The model under review builds one solid part; all positions refer to its coordinate system, in mm. Face numbers are marked on the shaded views. A direction names the side the tool comes from. Round coordinates to 2 decimals unless told otherwise and drop trailing zeros. Order: outer loops, then holes, each group sorted by start corner. A loop starts at its lowest first (then second) coordinate and runs counter-clockwise, first axis right, second up.
1) Consider section C-C (y = 49). Give the boundary of the cut face in (x, z).
2) Mouldability with a two-part tool opening along X and no side actions: class the marked faces 3, 4 and 5 as pulls with the +X half, pulls with the -X half, needs draft (parallel to the pull), parting line crosses it, or undercut.
3) To check wall thickness, follow L1, parallel to X at y = 69, z = -373; L2, parallel to X at y = 66, z = 120.5; L3, parallel to Y at x = -150, z = 281. State the ranges of each line that lie inside material, in increasing order.
4) Consider section A-A (x = 88.51). Give the boundary of the cut face in (y, z), then the cut area to 3 significant figures.
5) Consider section B-B (z = -186.5). Give the boundary of the cut face in (x, y).
6) Machinability: for the marked faces 1 and 2, which of the approach directions +Z, -Z, +X, -X, +Y, -Y give a long, thin tool a straight path to every point of the face, cutting with its end or side? Answer none if there is none.
7) Clearance check with flat-ended pins moving along their axes: P1, Ø12, axis at x = -106.5, y = 73.5, coming from the +Z side; P2, Ø3, axis at x = 51.5, z = -3.5, coming from the -Y side; P3, Ø6, axis at x = 109.5, z = 313.5, coming from the -Y side; P4, Ø5, axis at x = 29.5, y = 18.5, coming from the +Z side. State where each tip first meets the part, or that it passes through.
8) Consider section D-D (x = 10). Give the boundary of the cut face in (y, z).
from build123d import *

# Parameters (mm, degrees)
BOSS_EXTRUDE1_DEPTH = 591.5
SKETCH2_W           = 388.02090207
SKETCH2_H           = 25.404192512
BOSS_EXTRUDE2_DEPTH = 232
FILLET1_R           = 12.7
FILLET3_R           = 6.35


with BuildPart() as part:
    # Sketch1 → Boss-Extrude1 (new body)
    with BuildSketch(Plane(origin=(0, 0, -411.75), x_dir=(-1, 0, 0), z_dir=(0, 0, -1))):
        with BuildLine():
            Line((121.01, 20.009665474), (194.010451035, 36.954192512))
            Line((194.010451035, 36.954192512), (194.010451035, 103.904192512))
            Line((194.010451035, 103.904192512), (-194.010451035, 103.904192512))
            Line((-194.010451035, 103.904192512), (-194.010451035, 36.954192512))
            Line((-194.010451035, 36.954192512), (-121.01, 20.009665474))
            Line((-121.01, 20.009665474), (-121.01, 39))
            ThreePointArc((-121.01, 39), (-88.51, 71.5), (-56.01, 39))
            Line((-56.01, 39), (-56.01, 5.206473282))
            ThreePointArc((-56.01, 5.206473282), (0, 0), (56.01, 5.206473282))
            Line((56.01, 5.206473282), (56.01, 39))
            ThreePointArc((56.01, 39), (88.51, 71.5), (121.01, 39))
            Line((121.01, 39), (121.01, 20.009665474))
        make_face()
    extrude(amount=-BOSS_EXTRUDE1_DEPTH)

    # Sketch2 → Boss-Extrude2 (add)
    with BuildSketch(Plane.XY.offset(179.75)):
        with Locations((0, 91.202096256)):
            Rectangle(SKETCH2_W, SKETCH2_H)
    extrude(amount=BOSS_EXTRUDE2_DEPTH)

    # Fillet1
    fillet1_edges = [part.edges().sort_by_distance(p)[0] for p in [
        (194.010451035, 70.429192512, -411.75),
        (-194.010451035, 70.429192512, -411.75),
        (194.010451035, 91.202096256, 411.75),
        (-194.010451035, 91.202096256, 411.75),
    ]]
    fillet(fillet1_edges, radius=FILLET1_R)

    # Fillet3
    fillet3_edges = [part.edges().sort_by_distance(p)[0] for p in [
        (0, 78.5, 179.75),
    ]]
    fillet(fillet3_edges, radius=FILLET3_R)


solid = part.part
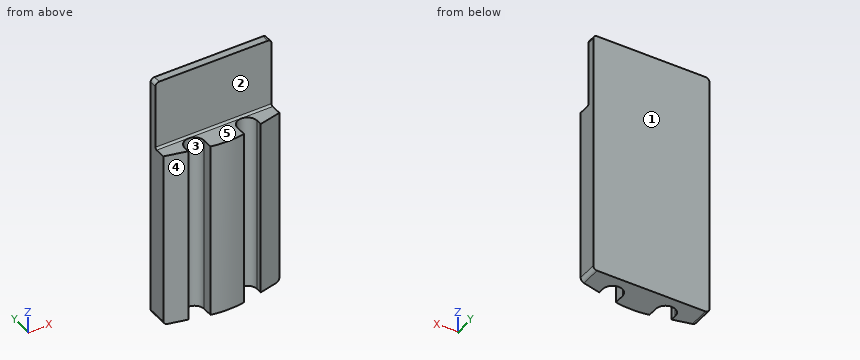
Answer below:
1. outline: (-194.01, -399.05) arc R12.7 ccw to (-181.31, -411.75) - (-119.43, -411.75) - (-119.43, 179.75) - (-194.01, 179.75) - close; (-57.59, -411.75) - (57.59, -411.75) - (57.59, 179.75) - (-57.59, 179.75) - close; (119.43, -411.75) - (181.31, -411.75) arc R12.7 ccw to (194.01, -399.05) - (194.01, 179.75) - (119.43, 179.75) - close
2. face 3: undercut
2. face 4: pulls with the -X half
2. face 5: needs draft
3. L1: x = -194.01 to -101.01, -76.01 to 76.01, 101.01 to 194.01
3. L2: x = -194.01 to -106.6, -70.42 to 70.42, 106.6 to 194.01
3. L3: y = 78.5 to 103.9
4. outline: (71.5, -411.75) - (103.9, -411.75) - (103.9, 411.75) - (78.5, 411.75) - (78.5, 186.1) arc R6.35 cw to (72.15, 179.75) - (71.5, 179.75) - close
4. area: 25,100 mm2
5. outline: (-194.01, 36.95) - (-121.01, 20.01) - (-121.01, 39) arc R32.5 cw to (-56.01, 39) - (-56.01, 5.21) arc R303.87 ccw to (56.01, 5.21) - (56.01, 39) arc R32.5 cw to (121.01, 39) - (121.01, 20.01) - (194.01, 36.95) - (194.01, 103.9) - (-194.01, 103.9) - close
6. face 1: +Z, -Z, +X, -X, +Y
6. face 2: +Z, +X, -X, -Y
7. P1: stops at z = 411.75
7. P2: stops at y = 4.14
7. P3: stops at y = 78.5
7. P4: stops at z = 179.75
8. outline: (0.16, -411.75) - (103.9, -411.75) - (103.9, 411.75) - (78.5, 411.75) - (78.5, 186.1) arc R6.35 cw to (72.15, 179.75) - (0.16, 179.75) - close
